from build123d import *

# Parameters (mm, degrees)
BOSS_EXTRU_1_DEPTH      = 20
CONG_1_R                = 10
CONG_2_R                = 10
CONG_3_R                = 10
CONG_4_R                = 10
CONG_5_R                = 10
CONG_7_R                = 10
ESQUISSE2_W             = 20
ESQUISSE2_H             = 120
BOSS_EXTRU_2_DEPTH      = 130
CONG_8_R                = 60
CONG_9_R                = 60
CONG_10_R               = 60
CONG_11_R               = 60
ESQUISSE3_R             = 35
ENL_V_MAT_EXTRU_1_DEPTH = 258.77353424
ESQUISSE4_R             = 9
ENL_V_MAT_EXTRU_2_DEPTH = 335.555805948
ESQUISSE5_R             = 19.375511008
ESQUISSE5_R_2           = 19.500884668
ENL_V_MAT_EXTRU_3_DEPTH = 3


with BuildPart() as part:
    # Esquisse1 → Boss.-Extru.1 (new body)
    with BuildSketch(Plane.XY):
        Polygon((-254.799934421, 65.838280942), (-298.101203362, -9.161719058), (-254.799931925, -84.161719058), (-94.799931925, -84.161719058), (-51.498662984, -9.161719058), (-94.799934421, 65.838280942), align=None)
    extrude(amount=BOSS_EXTRU_1_DEPTH)

    # Congé1
    cong_1_edges = [part.edges().sort_by_distance(p)[0] for p in [
        (-94.799934421, 65.838280942, 10),
    ]]
    fillet(cong_1_edges, radius=CONG_1_R)

    # Congé2
    cong_2_edges = [part.edges().sort_by_distance(p)[0] for p in [
        (-254.799934421, 65.838280942, 10),
    ]]
    fillet(cong_2_edges, radius=CONG_2_R)

    # Congé3
    cong_3_edges = [part.edges().sort_by_distance(p)[0] for p in [
        (-298.101203362, -9.161719058, 10),
    ]]
    fillet(cong_3_edges, radius=CONG_3_R)

    # Congé4
    cong_4_edges = [part.edges().sort_by_distance(p)[0] for p in [
        (-254.799931925, -84.161719058, 10),
    ]]
    fillet(cong_4_edges, radius=CONG_4_R)

    # Congé5
    cong_5_edges = [part.edges().sort_by_distance(p)[0] for p in [
        (-94.799931925, -84.161719058, 10),
    ]]
    fillet(cong_5_edges, radius=CONG_5_R)

    # Congé7
    cong_7_edges = [part.edges().sort_by_distance(p)[0] for p in [
        (-51.498662984, -9.161719058, 10),
    ]]
    fillet(cong_7_edges, radius=CONG_7_R)

    # Esquisse2 → Boss.-Extru.2 (add)
    with BuildSketch(Plane.XY.offset(20)):
        with Locations((-234.554197979, -9.161719058)):
            Rectangle(ESQUISSE2_W, ESQUISSE2_H)
        with Locations((-114.554197979, -9.161719058)):
            Rectangle(ESQUISSE2_W, ESQUISSE2_H)
    extrude(amount=BOSS_EXTRU_2_DEPTH)

    # Congé8
    cong_8_edges = [part.edges().sort_by_distance(p)[0] for p in [
        (-114.554197979, -69.161719058, 150),
    ]]
    fillet(cong_8_edges, radius=CONG_8_R)

    # Congé9
    cong_9_edges = [part.edges().sort_by_distance(p)[0] for p in [
        (-114.554197979, 50.838280942, 150),
    ]]
    fillet(cong_9_edges, radius=CONG_9_R - 0.0001)  # a hair under: the kernel refuses the full size

    # Congé10
    cong_10_edges = [part.edges().sort_by_distance(p)[0] for p in [
        (-234.554197979, -69.161719058, 150),
    ]]
    fillet(cong_10_edges, radius=CONG_10_R)

    # Congé11
    cong_11_edges = [part.edges().sort_by_distance(p)[0] for p in [
        (-234.554197979, 50.838280942, 150),
    ]]
    fillet(cong_11_edges, radius=CONG_11_R - 0.0001)  # a hair under: the kernel refuses the full size

    # Esquisse3 → Enlèv. mat.-Extru.1 (cut, through all)
    with BuildSketch(Plane(origin=(-104.554197979, 0, 0), x_dir=(0, 0, -1), z_dir=(1, 0, 0))):
        with Locations(Location((-90, -9.161719058, 0), (0, 0, 90))):
            Circle(ESQUISSE3_R)
    extrude(amount=-ENL_V_MAT_EXTRU_1_DEPTH, mode=Mode.SUBTRACT)

    # Esquisse4 → Enlèv. mat.-Extru.2 (cut, through all)
    with BuildSketch(Plane.XY.offset(20)):
        with Locations((-274.554197979, -9.161719058)):
            Circle(ESQUISSE4_R)
        with Locations((-75.045668368, -9.161719084)):
            Circle(ESQUISSE4_R)
    extrude(amount=-ENL_V_MAT_EXTRU_2_DEPTH, mode=Mode.SUBTRACT)

    # Esquisse5 → Enlèv. mat.-Extru.3 (cut)
    with BuildSketch(Plane.XY.offset(20)):
        with Locations((-274.554197979, -9.161719058)):
            Circle(ESQUISSE5_R)
        with Locations((-75.045668368, -9.161719084)):
            Circle(ESQUISSE5_R_2)
    extrude(amount=-ENL_V_MAT_EXTRU_3_DEPTH, mode=Mode.SUBTRACT)


solid = part.part
Input: part model. Units: mm. Frame: model coordinates. A direction names the side the tool comes from. Coordinates: 2 decimals unless noted, no trailing zeros. Write each loop counter-clockwise with the first axis right and the second up, starting at its lowest first coordinate (ties: lowest second). Pieces come first, ordered by that corner, then holes. Notation, with made-up numbers: M -3.5,14.5 L 35.5,14.5 A26 ccw 35.5,42.5 Z; hole C 86,41.5 d3. An arc over 180 degrees is marked long. Answer as a JSON object with one key per item and string values. Group by question number.
(1) Contact query for flat-ended pins moving along their axis: P1, Ø19.5, axis at x = -275, y = -2.5, coming from the +Z side; P2, Ø6, axis at x = -243.5, z = 35.5, coming from the +Y side; P3, Ø10, axis at x = -113.5, z = 43, coming from the -Y side. Output: stop coordinate, or through.
(2) Section C-C on z = 116. Output: boundary loops of the cut face in (x, y).
(3) Section A-A on y = 4.5. Output: boundary loops of the cut face in (x, z), plus the area to 3 significant figures.
(4) Mould query, pull axis Y, two halves, no side actions, for faces 1 (the face through (-281.696, -14.638, 8.619)), 2 (the face through (-244.554, -23, 55)), 3 (the face through (-115, 50.838, 55)), 4 (the face through (-66.7, -13.2, 17)). Classes: pulls with the +Y half, pulls with the -Y half, needs draft (parallel to the pull), parting line crosses it, or undercut.
(5) Set-up query: faces 5 (the face through (-224.554, -23, 55)), 6 (the face through (-276.19, 28.79, 9.86)), 7 (the face through (-104.554, -23, 55)), 8 (the face through (-234.41, -52.05, 131.96)), 9 (the face through (-266, -13, 17)). Return all of +Z, -Z, +X, -X, +Y, -Y with unobstructed straight access to the full face (end or side cutting, diameter ignored); none if empty.
(6) Section D-D on x = -150.5. Output: boundary loops of the cut face in (y, z).
(7) Ray query, line 1 along X through (y, z) = (42, 117); line 2 along Y through (x, z) = (-233, 42.5); line 3 along Z through (x, y) = (-153, 23.5). Return the intervals inside material, ascending. Write a range as [from, to].
(8) Section B-B on z = 43.5. Output: boundary loops of the cut face in (x, y).
Result set:
{
 "1": {"P1": "stops at z = 17", "P2": "stops at y = 50.84", "P3": "stops at y = -69.16"},
 "2": {"outline": "M -244.55,-63.24 L -224.55,-63.24 L -224.55,-32.59 L -244.55,-32.59 Z; M -244.55,14.27 L -224.55,14.27 L -224.55,44.91 L -244.55,44.91 Z; M -124.55,-63.24 L -104.55,-63.24 L -104.55,-32.59 L -124.55,-32.59 Z; M -124.55,14.27 L -104.55,14.27 L -104.55,44.91 L -124.55,44.91 Z"},
 "3": {"outline": "M -290.21,0 L -59.39,0 L -59.39,20 L -61.13,20 L -61.13,17 L -88.96,17 L -88.96,20 L -104.55,20 L -104.55,57.78 L -124.55,57.78 L -124.55,20 L -224.55,20 L -224.55,57.78 L -244.55,57.78 L -244.55,20 L -260.81,20 L -260.81,17 L -288.29,17 L -288.29,20 L -290.21,20 Z; M -244.55,122.22 L -224.55,122.22 L -224.55,148.42 L -244.55,148.42 Z; M -124.55,122.22 L -104.55,122.22 L -104.55,148.42 L -124.55,148.42 Z", "area": "7,010 mm2"},
 "4": {"face 1": "undercut", "face 2": "needs draft", "face 3": "pulls with the +Y half", "face 4": "undercut"},
 "5": {"face 5": "+Z, +Y, -Y", "face 6": "+Z, -Z, -X, +Y", "face 7": "+Z, +X, +Y, -Y", "face 8": "+Z, +X, -X, -Y", "face 9": "+Z"},
 "6": {"outline": "M -84.16,0 L 65.84,0 L 65.84,20 L -84.16,20 Z"},
 "7": {"line 1": "x = [-244.55, -224.55], [-124.55, -104.55]", "line 2": "y = [-69.16, 50.84]", "line 3": "z = [0, 20]"},
 "8": {"outline": "M -244.55,-69.16 L -224.55,-69.16 L -224.55,50.84 L -244.55,50.84 Z; M -124.55,-69.16 L -104.55,-69.16 L -104.55,50.84 L -124.55,50.84 Z"}
}
